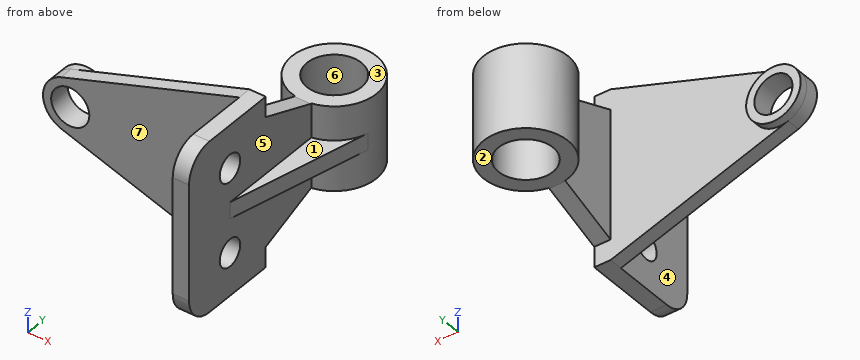
```python
from build123d import *
from build123d.topology import SkipClean

# Parameters (mm, degrees)
BOSS_EXTRUDE1_DEPTH      = 10
SKETCH2_R                = 20
BOSS_EXTRUDE2_DEPTH      = 6
CUT_EXTRUDE1_REACH       = 170.814
SKETCH3_R                = 14
BOSS_EXTRUDE3_DEPTH      = 31
BOSS_EXTRUDE3_DEPTH_BACK = 31
SKETCH4_R                = 31
SKETCH4_R_2              = 20
BOSS_EXTRUDE4_DEPTH      = 12
SKETCH7_R                = 10
BOSS_EXTRUDE5_DEPTH      = 12
BOSS_EXTRUDE6_DEPTH      = 6
BOSS_EXTRUDE6_DEPTH_BACK = 6


with BuildPart() as part:
    # Sketch1 → Boss-Extrude1 (new body)
    with BuildSketch(Plane(origin=(0, 0, 0), x_dir=(1, 0, 0), z_dir=(0, 1, 0))):
        with BuildLine():
            Line((0, 0), (0, -62.5))
            Line((0, -62.5), (-12, -62.5))
            Line((-12, -62.5), (-142.957379404, -18.750863229))
            ThreePointArc((-142.957379404, -18.750863229), (-155.997283991, 0.329595189), (-142.335664896, 18.969959154))
            Line((-142.335664896, 18.969959154), (-12, 62.5))
            Line((-12, 62.5), (0, 62.5))
            Line((0, 62.5), (0, 0))
        make_face()
    extrude(amount=BOSS_EXTRUDE1_DEPTH)

    # Sketch2 → Boss-Extrude2 (add)
    with BuildSketch(Plane(origin=(0, 10, 0), x_dir=(1, 0, 0), z_dir=(0, 1, 0))):
        with Locations(Location((-136, 0, 0), (0, 0, 108.468500272))):
            Circle(SKETCH2_R)
    extrude(amount=BOSS_EXTRUDE2_DEPTH)

    # Sketch3 → Cut-Extrude1 (cut, up to next)
    with BuildSketch(Plane(origin=(0, 16, 0), x_dir=(1, 0, 0), z_dir=(0, 1, 0)), mode=Mode.PRIVATE) as cut_extrude1_sk1:
        with Locations(Location((-136, 0, 0), (0, 0, 270))):
            Circle(SKETCH3_R)
    cut_extrude1_tool1 = extrude(cut_extrude1_sk1.sketch, amount=-CUT_EXTRUDE1_REACH, mode=Mode.PRIVATE) & part.part
    add(cut_extrude1_tool1.solids().sort_by_distance((-136, 16, 0))[0], mode=Mode.SUBTRACT)

    # Sketch5 → Boss-Extrude4 (add)
    with BuildSketch(Plane(origin=(0, 0, 0), x_dir=(0, 0, -1), z_dir=(1, 0, 0))):
        Polygon((-47.5, 10), (-31, 54), (-31, 60.618293766), (31, 60.618293766), (31, 54), (47.5, 10), align=None)
    extrude(amount=-BOSS_EXTRUDE4_DEPTH)

    # Sketch7 → Boss-Extrude5 (add)
    with SkipClean():  # the faces are left unmerged after this step: merging them gives an invalid solid
        with BuildSketch(Plane(origin=(0, 0, 0), x_dir=(0, 0, -1), z_dir=(1, 0, 0))):
            with BuildLine():
                Line((-62.5, 0), (-62.5, -45))
                ThreePointArc((-62.5, -45), (-56.642135624, -59.142135624), (-42.5, -65))
                Line((-42.5, -65), (42.5, -65))
                ThreePointArc((42.5, -65), (56.642135624, -59.142135624), (62.5, -45))
                Line((62.5, -45), (62.5, 0))
                Line((62.5, 0), (-62.5, 0))
            make_face()
            with Locations((-31, -25)):
                Circle(SKETCH7_R, mode=Mode.SUBTRACT)
            with Locations((31, -25)):
                Circle(SKETCH7_R, mode=Mode.SUBTRACT)
        extrude(amount=-BOSS_EXTRUDE5_DEPTH)



with BuildPart() as body_2:
    # Sketch4 → Boss-Extrude3 (new, two sides: drawn at the far end of the back side and taken through both)
    with BuildSketch(Plane.XY.offset(-BOSS_EXTRUDE3_DEPTH_BACK)):
        with Locations((-6, 85)):
            Circle(SKETCH4_R)
        with Locations((-6, 85)):
            Circle(SKETCH4_R_2, mode=Mode.SUBTRACT)
    extrude(amount=BOSS_EXTRUDE3_DEPTH + BOSS_EXTRUDE3_DEPTH_BACK)


with BuildPart() as part_1:
    with SkipClean():  # the faces are left unmerged after this step: merging them gives an invalid solid
        add(part.part)

        add(body_2.part)  # Boss-Extrude6 merges body 2
        # Sketch8 → Boss-Extrude6 (add, two sides: drawn at the far end of the back side and taken through both)
        with BuildSketch(Plane.XY.offset(-BOSS_EXTRUDE6_DEPTH_BACK)):
            with BuildLine():
                Line((0, -25), (24.178270058, 77.909723821))
                ThreePointArc((24.178270058, 77.909723821), (15.52239867, 62.688873729), (0, 54.586187349))
                Line((0, 54.586187349), (0, -25))
            make_face()
        extrude(amount=BOSS_EXTRUDE6_DEPTH + BOSS_EXTRUDE6_DEPTH_BACK)


solid = part_1.part
```
Verification items for the finished model (mm, model axes). Face numbers are marked on the shaded views. A direction names the side the tool comes from. Coordinates: 2 decimals unless noted, no trailing zeros. Loops run counter-clockwise (first coordinate to the right, second up) from the corner with the lowest first, then second, coordinate; pieces in that order, holes last. Notation, with made-up numbers: (-18.5, 78.5) - (-1.5, 78.5) arc R9 cw to (-1.5, 91.5) - close; hole circle Ø5 at (-19, 52). An arc over 180 degrees is marked (long way). Put each result on its own line as item: value.
Item 1: Draft check along Y on the marked faces 5, 6 and 7. Enter one of: pulls with the +Y half, pulls with the -Y half, needs draft (parallel to the pull), parting line crosses it, or undercut.
Conclusion:
face 5: needs draft
face 6: undercut
face 7: pulls with the -Y half
Item 2: Section check D-D (x = -136). Enter the section's corners in (y, z), then the cut area to 3 significant figures.
Conclusion:
outline: (0, -21.09) - (10, -21.09) - (10, -20) - (16, -20) - (16, -14) - (0, -14) - close; (0, 14) - (16, 14) - (16, 20) - (10, 20) - (10, 21.08) - (0, 21.08) - close
area: 214 mm2
Item 3: Scan lines: line 1 along X through (y, z) = (-42, -53); line 2 along Y through (x, z) = (-101, -26.5); line 3 along Y through (x, z) = (-6, -11). Record each from-to range of solid material in increasing order.
Conclusion:
line 1: x = -12 to 0
line 2: y = 0 to 10
line 3: y = -65 to 65, 105 to 116
Item 4: Set-up check for the marked faces 1, 2, 3 and 4: record each of +Z, -Z, +X, -X, +Y, -Y from which the full face is reachable in a straight line by a thin tool's end or side.
Conclusion:
face 1: +Z, +X, -Y
face 2: -Z, +X, -X, +Y
face 3: +Z, +X, -X, +Y
face 4: +Z, -Z, -X, -Y
Item 5: Section check A-A (y = 85). Enter the section's corners in (x, z), then the cut area to 3 significant figures.
Conclusion:
outline: (-37, -31) - (-26, -31) - (-26, 31) - (-37, 31) - close; (14, -31) - (25, -31) - (25, 31) - (14, 31) - close
area: 1,360 mm2
Item 6: Section check B-B (x = -7.5). Enter the section's corners in (y, z).
Conclusion:
outline: (-65, -42.5) arc R20 ccw to (-45, -62.5) - (10, -62.5) - (10, -47.5) - (54, -31) - (65.06, -31) - (65.06, 31) - (54, 31) - (10, 47.5) - (10, 62.5) - (-45, 62.5) arc R20 ccw to (-65, 42.5) - close; (104.94, -31) - (115.96, -31) - (115.96, 31) - (104.94, 31) - close; hole circle Ø20 at (-25, -31); hole circle Ø20 at (-25, 31)
Item 7: Gauge pin test, flat ends, axial feed: pin 1 Ø6 at (x, z) = (-82.5, 16.5) entering from +Y; pin 2 Ø1.5 at (y, z) = (-5, 35) entering from -X; pin 3 Ø2 at (y, z) = (28.5, 18.5) entering from +X; pin 4 Ø18.5 at (x, y) = (-4.5, 86.5) entering from -Z. Record the tip position at first contact, or that the pin passes through.
Conclusion:
pin 1: stops at y = 10
pin 2: stops at x = -12
pin 3: stops at x = 0
pin 4: passes through
Item 8: Section check C-C (y = -20). Enter the section's corners in (x, z).
Conclusion:
outline: (-12, -62.5) - (0, -62.5) - (0, -39.66) - (-12, -39.66) - close; (-12, -22.34) - (0, -22.34) - (0, -6) - (1.17, -6) - (1.17, 6) - (0, 6) - (0, 22.34) - (-12, 22.34) - close; (-12, 39.66) - (0, 39.66) - (0, 62.5) - (-12, 62.5) - close
